Build history of the part. All positions in model axes, mm. A direction names the side the tool comes from. Give positions to 0.01 mm unless a question says otherwise; leave off trailing zeros. Order: outer loops, then holes, each group sorted by start corner. A loop starts at its lowest first (then second) coordinate and runs counter-clockwise, first axis right, second up. Notation, with made-up numbers: (30, 64.25) -> (54, 64.25) arc R29 ccw to (54, 95.25) -> close; hole circle Ø2 at (-9, -26). An arc over 180 degrees is marked (long way). Use a Markdown table: item, result. Add a question column.
```python
from build123d import *

# Parameters (mm, degrees)
SZKIC1_R                    = 5.25
DODANIE_WYCI_GNI_CIE1_DEPTH = 61.5
SZKIC3_R                    = 3.35
DODANIE_WYCI_GNI_CIE2_DEPTH = 8
SZKIC4_R                    = 2.5
WYTNIJ_WYCI_GNI_CIE2_DEPTH  = 70.5
SZKIC7_R                    = 3.05
WYTNIJ_WYCI_GNI_CIE4_DEPTH  = 18
WYTNIJ_WYCI_GNI_CIE8_DEPTH  = 8


with BuildPart() as part:
    # Szkic1 → Dodanie-wyciągnięcie1 (new body)
    with BuildSketch(Plane.XY):
        Circle(SZKIC1_R)
    extrude(amount=DODANIE_WYCI_GNI_CIE1_DEPTH)

    # Szkic3 → Dodanie-wyciągnięcie2 (add)
    with BuildSketch(Plane.XY.offset(61.5)):
        Circle(SZKIC3_R)
    extrude(amount=DODANIE_WYCI_GNI_CIE2_DEPTH)

    # Szkic4 → Wytnij-wyciągnięcie2 (cut, through all)
    with BuildSketch(Plane.XY.offset(69.5)):
        Circle(SZKIC4_R)
    extrude(amount=-WYTNIJ_WYCI_GNI_CIE2_DEPTH, mode=Mode.SUBTRACT)

    # Szkic7 → Wytnij-wyciągnięcie4 (cut)
    with BuildSketch(Plane(origin=(0, 0, 0), x_dir=(-1, 0, 0), z_dir=(0, 0, -1))):
        Circle(SZKIC7_R)
    extrude(amount=-WYTNIJ_WYCI_GNI_CIE4_DEPTH, mode=Mode.SUBTRACT)

    # Szkic10 → Wytnij-wyciągnięcie8 (cut)
    with BuildSketch(Plane.XY.offset(69.5)):
        Polygon((-2.5, 4.616546328), (-2.45, 4.616546328), (-2.45, -4.155907231), (-2.5, -4.155907231), (-5.821141217, -4.155907231), (-5.821141217, 4.616546328), align=None)
        Polygon((2.5, 4.616546328), (2.45, 4.616546328), (2.45, -4.055418973), (2.5, -4.055418973), (5.892918543, -4.155907231), (5.892918543, 4.616546328), align=None)
    extrude(amount=-WYTNIJ_WYCI_GNI_CIE8_DEPTH, mode=Mode.SUBTRACT)


solid = part.part
```
(1) Mould opens along Y. For faces 6 (the face through (2.385, 0.751, 44.11)), 7 (the face through (5, 1.6, 30.3)), 8 (the face through (3.047, 0.134, 8.874)), 9 (the face through (-2.45, 1.4, 65.6)) say: released by +Y, released by -Y, zero draft, split by the parting line, or undercut.
(2) Band-saw the part on A-A on x = 0. Give the cut face in (y, z), plus the area to 3 significant figures.
(3) Pin check, flat tips, straight feed: pin 1 Ø2 at (x, y) = (4, 1) entering from -Z; pin 2 Ø1 at (y, z) = (2, 35.5) entering from -X; pin 3 Ø1 at (x, z) = (-4, 52.5) entering from -Y; pin 4 Ø2 at (y, z) = (-1.5, 63.5) entering from -X. Stop position of each tip, or through.
(4) Wall check: probe 1 along X at (y, z) = (0, 38); probe 2 along Y at (x, z) = (0, 14.25). Give the ranges that are in metal, low to high.
(5) Tool access for faces 1 (the face through (-0.04, -3.35, 65.44)), 2 (the face through (0.04, 3.35, 65.44)), 3 (the face through (-2.45, -1.4, 65.6)), 4 (the face through (3, 0, 61.5)), 5 (the face through (2.45, 1.4, 65.6)): list every direction of +Z, -Z, +X, -X, +Y, -Y with a clear straight run to the whole face (end or side of a thin tool).
(6) Band-saw the part on D-D on y = 4. Give the cut face in (x, z).
(7) Band-saw the part on C-C on z = 22.5. Give the cut face in (x, y), plus the area to 3 significant figures.
(8) Band-saw the part on B-B on y = -1.25. Give the cut face in (x, z).
Response:
| question | item | result |
|---|---|---|
| 1 | face 6 | undercut |
| 1 | face 7 | split by the parting line |
| 1 | face 8 | undercut |
| 1 | face 9 | zero draft |
| 2 | outline | (-5.25, 0) -> (-3.05, 0) -> (-3.05, 18) -> (-2.5, 18) -> (-2.5, 69.5) -> (-3.35, 69.5) -> (-3.35, 61.5) -> (-5.25, 61.5) -> close; (2.5, 18) -> (3.05, 18) -> (3.05, 0) -> (5.25, 0) -> (5.25, 61.5) -> (3.35, 61.5) -> (3.35, 69.5) -> (2.5, 69.5) -> close |
| 2 | area | 332 mm² |
| 3 | pin 1 | stops at z = 0 |
| 3 | pin 2 | stops at x = -5.03 |
| 3 | pin 3 | stops at y = -3.91 |
| 3 | pin 4 | stops at x = -2.45 |
| 4 | probe 1 | x = -5.25 to -2.5, 2.5 to 5.25 |
| 4 | probe 2 | y = -5.25 to -3.05, 3.05 to 5.25 |
| 5 | face 1 | +Z, -Y |
| 5 | face 2 | +Z, +Y |
| 5 | face 3 | +Z, -X, +Y, -Y |
| 5 | face 4 | +Z |
| 5 | face 5 | +Z, +X, +Y, -Y |
| 6 | outline | (-3.4, 0) -> (3.4, 0) -> (3.4, 61.5) -> (-3.4, 61.5) -> close |
| 7 | outline | circle Ø10.5 at (0, 0); hole circle Ø5 at (0, 0) |
| 7 | area | 67.0 mm² |
| 8 | outline | (-5.1, 0) -> (-2.78, 0) -> (-2.78, 18) -> (-2.17, 18) -> (-2.17, 69.5) -> (-2.45, 69.5) -> (-2.45, 61.5) -> (-5.1, 61.5) -> close; (2.17, 18) -> (2.78, 18) -> (2.78, 0) -> (5.1, 0) -> (5.1, 61.5) -> (2.45, 61.5) -> (2.45, 69.5) -> (2.17, 69.5) -> close |
